Input: part model. Units: mm. Frame: model coordinates. Face numbers are marked on the shaded views. A direction names the side the tool comes from. Round coordinates to 2 decimals unless told otherwise and drop trailing zeros. Loops run counter-clockwise (first coordinate to the right, second up) from the corner with the lowest first, then second, coordinate; pieces in that order, holes last. Notation, with made-up numbers: M 34,-29.75 L 69,-29.75 A15 ccw 69,-14.75 Z; hole C 39.5,42.5 d8. An arc over 180 degrees is marked long. Return JSON: item names as keys, results as strings. Group by question number.
1) Section B-B (y = 41). Output: boundary loops of the cut face in (x, z).
2) Access query for the marked faces 4, 5, 6, 7 and 8. Directions: +Z, -Z, +X, -X, +Y, -Y. A direction counts if a zero-diameter tool reaches every point of the face in a straight line with its end or side. Return the directions, or none.
3) Section C-C (y = 31). Output: boundary loops of the cut face in (x, z), plus the area to 3 significant figures.
4) Mould query, pull axis X, two halves, no side actions, for the marked faces 1, 2 and 3. Classes: +X half, -X half, draft (parallel to the pull), parting line (faces both ways), or undercut.
5) Section A-A (x = 30.5). Count the separate pieces of the cut face and the enclosed holes in it, plus the area to 3 significant figures.
6) Contact query for flat-ended pins moving along their axis: P1, Ø10, axis at x = 42, z = -5.5, coming from the -Y side; P2, Ø1.5, axis at x = 17, y = 32.5, coming from the -Z side; P3, Ø5, axis at x = 20, z = 1, coming from the +Y side. Output: stop coordinate, or through.
7) Material intervals for line 1 (X direction, y = 21, z = -0.75); line 2 (Y direction, x = 11.5, z = -7.75); line 3 (Z direction, x = 47, y = 21.5), sorted ascending. Write a range as from..to.
8) Section D-D (y = -1). Output: boundary loops of the cut face in (x, z).
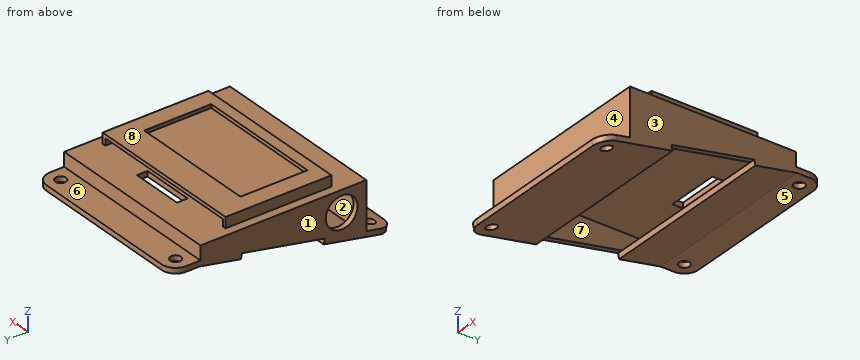
from build123d import *

# Parameters (mm, degrees)
SKETCH_1_W          = 51
SKETCH_1_H          = 47
SKETCH_1_W_2        = 15
SKETCH_1_H_2        = 3
EXTRUDE_1_DEPTH     = 1.5
EXTRUDE_2_DEPTH     = 2
SKETCH_3_W          = 46
SKETCH_3_H          = 30
SKETCH_3_W_2        = 36
SKETCH_3_H_2        = 19
EXTRUDE_3_DEPTH     = 1
SKETCH_4_W          = 51
SKETCH_4_H          = 47
SKETCH_4_W_2        = 48
SKETCH_4_H_2        = 44.5
EXTRUDE_4_DEPTH     = 12
CUT_EXTRUDE_1_DEPTH = 52
SKETCH_6_W          = 51
SKETCH_6_H          = 12
SKETCH_6_R          = 1.5
EXTRUDE_5_DEPTH     = 1.5
SKETCH_7_W          = 1.5
SKETCH_7_H          = 8
EXTRUDE_6_DEPTH     = 51
FILLET_1_R          = 4
CUT_EXTRUDE_2_REACH = 14.585
SKETCH_8_R          = 1.5
CUT_EXTRUDE_3_REACH = 53
SKETCH_9_R          = 4.5


with BuildPart() as part:
    # 草图1 → 凸台-拉伸1 (new body)
    with BuildSketch(Plane.XY):
        with Locations((25.5, 23.5)):
            Rectangle(SKETCH_1_W, SKETCH_1_H)
        with Locations((25.5, 38.5)):
            Rectangle(SKETCH_1_W_2, SKETCH_1_H_2, mode=Mode.SUBTRACT)
    extrude(amount=EXTRUDE_1_DEPTH)

    # 草图2 → 凸台-拉伸2 (add)
    with BuildSketch(Plane.XY.offset(1.5)):
        Polygon((2.5, 8), (48.5, 8), (48.5, 38), (47.5, 38), (47.5, 9), (3.5, 9), (3.5, 38), (2.5, 38), align=None)
    extrude(amount=EXTRUDE_2_DEPTH)

    # 草图3 → 凸台-拉伸3 (add)
    with BuildSketch(Plane.XY.offset(3.5)):
        with Locations((25.5, 23)):
            Rectangle(SKETCH_3_W, SKETCH_3_H)
        with Locations((25.5, 20.5)):
            Rectangle(SKETCH_3_W_2, SKETCH_3_H_2, mode=Mode.SUBTRACT)
    extrude(amount=EXTRUDE_3_DEPTH)

    # 草图4 → 凸台-拉伸4 (add)
    with BuildSketch(Plane(origin=(0, 0, 0), x_dir=(-1, 0, 0), z_dir=(0, 0, -1))):
        with Locations((-25.5, 23.5)):
            Rectangle(SKETCH_4_W, SKETCH_4_H)
        with Locations((-25.5, 23.75)):
            Rectangle(SKETCH_4_W_2, SKETCH_4_H_2, mode=Mode.SUBTRACT)
    extrude(amount=EXTRUDE_4_DEPTH)

    # 草图5 → 切除-拉伸1 (cut, through all)
    with BuildSketch(Plane(origin=(51, 0, 0), x_dir=(0, 0, -1), z_dir=(1, 0, 0))):
        Polygon((2.5, 47), (12, 47), (12, 0), align=None)
    extrude(amount=-CUT_EXTRUDE_1_DEPTH, mode=Mode.SUBTRACT)

    # 草图6 → 凸台-拉伸5 (add)
    with BuildSketch(Plane(origin=(0, 2.330325106, -11.52897684), x_dir=(-1, 0, 0), z_dir=(0, 0.198120998, -0.980177571))):
        with Locations((-25.5, 39.573043325)):
            Rectangle(SKETCH_6_W, SKETCH_6_H)
        with BuildLine():
            Line((-51, 9.62254802), (0, 9.62254802))
            Line((0, 9.62254802), (0, -6.37745198))
            ThreePointArc((0, -6.37745198), (-1.171572875, -9.205879105), (-4, -10.37745198))
            Line((-4, -10.37745198), (-47, -10.37745198))
            ThreePointArc((-47, -10.37745198), (-49.828427125, -9.205879105), (-51, -6.37745198))
            Line((-51, -6.37745198), (-51, 9.62254802))
        make_face()
        with Locations((-47, -6.37745198)):
            Circle(SKETCH_6_R, mode=Mode.SUBTRACT)
        with Locations((-4, -6.37745198)):
            Circle(SKETCH_6_R, mode=Mode.SUBTRACT)
    extrude(amount=EXTRUDE_5_DEPTH)

    # 草图7 → 凸台-拉伸6 (add)
    with BuildSketch(Plane(origin=(51, 0, 0), x_dir=(0, 0, -1), z_dir=(1, 0, 0))):
        with Locations((3.220266356, 51)):
            Rectangle(SKETCH_7_W, SKETCH_7_H)
    extrude(amount=-EXTRUDE_6_DEPTH)

    # 圆角1
    fillet_1_edges = [part.edges().sort_by_distance(p)[0] for p in [
        (51, 55, -3.220266356),
        (0, 55, -3.220266356),
    ]]
    fillet(fillet_1_edges, radius=FILLET_1_R)

    # 草图8 → 切除-拉伸2 (cut, up to next)
    with BuildSketch(Plane.XY.offset(-2.470266356), mode=Mode.PRIVATE) as cut_extrude_2_sk1:
        with Locations((4, 51)):
            Circle(SKETCH_8_R)
    cut_extrude_2_tool1 = extrude(cut_extrude_2_sk1.sketch, amount=-CUT_EXTRUDE_2_REACH, mode=Mode.PRIVATE) & part.part
    add(cut_extrude_2_tool1.solids().sort_by_distance((4, 51, -2.470266))[0], mode=Mode.SUBTRACT)
    # 草图8 → 切除-拉伸2 (cut, up to next)
    with BuildSketch(Plane.XY.offset(-2.470266356), mode=Mode.PRIVATE) as cut_extrude_2_sk2:
        with Locations((47, 51)):
            Circle(SKETCH_8_R)
    cut_extrude_2_tool2 = extrude(cut_extrude_2_sk2.sketch, amount=-CUT_EXTRUDE_2_REACH, mode=Mode.PRIVATE) & part.part
    add(cut_extrude_2_tool2.solids().sort_by_distance((47, 51, -2.470266))[0], mode=Mode.SUBTRACT)

    # 草图9 → 切除-拉伸3 (cut, up to next)
    with BuildSketch(Plane.ZY, mode=Mode.PRIVATE) as cut_extrude_3_sk1:
        with Locations((-4.5, 7)):
            Circle(SKETCH_9_R)
    cut_extrude_3_tool1 = extrude(cut_extrude_3_sk1.sketch, amount=-CUT_EXTRUDE_3_REACH, mode=Mode.PRIVATE) & part.part
    add(cut_extrude_3_tool1.solids().sort_by_distance((0, 7, -4.5))[0], mode=Mode.SUBTRACT)


solid = part.part
Returned:
{
 "1": {"outline": "M 0,-5.24 L 51,-5.24 L 51,1.5 L 0,1.5 Z; hole M 1.5,-3.71 L 49.5,-3.71 L 49.5,0 L 1.5,0 Z"},
 "2": {"face 4": "+Z, +X, -X, -Y", "face 5": "-Z, +X, -X, +Y", "face 6": "+Z, +X, -X, +Y", "face 7": "none", "face 8": "+Z, +X, -X, +Y, -Y"},
 "3": {"outline": "M 0,-5.73 L 1.5,-5.73 L 1.5,0 L 49.5,0 L 49.5,-5.73 L 51,-5.73 L 51,1.5 L 48.5,1.5 L 48.5,4.5 L 2.5,4.5 L 2.5,1.5 L 0,1.5 Z; hole M 3.5,1.5 L 47.5,1.5 L 47.5,3.5 L 3.5,3.5 Z", "area": "144 mm^2"},
 "4": {"face 1": "-X half", "face 2": "undercut", "face 3": "+X half"},
 "5": {"separate pieces": "3", "enclosed holes": "0", "area": "159 mm^2"},
 "6": {"P1": "stops at y = 0", "P2": "stops at z = 0", "P3": "stops at y = 47"},
 "7": {"line 1": "x = 0..1.5, 49.5..51", "line 2": "y = 0..1.5", "line 3": "z = 0..1.5, 3.5..4.5"},
 "8": {"outline": "M 0,-13.73 L 51,-13.73 L 51,-12.2 L 0,-12.2 Z"}
}
